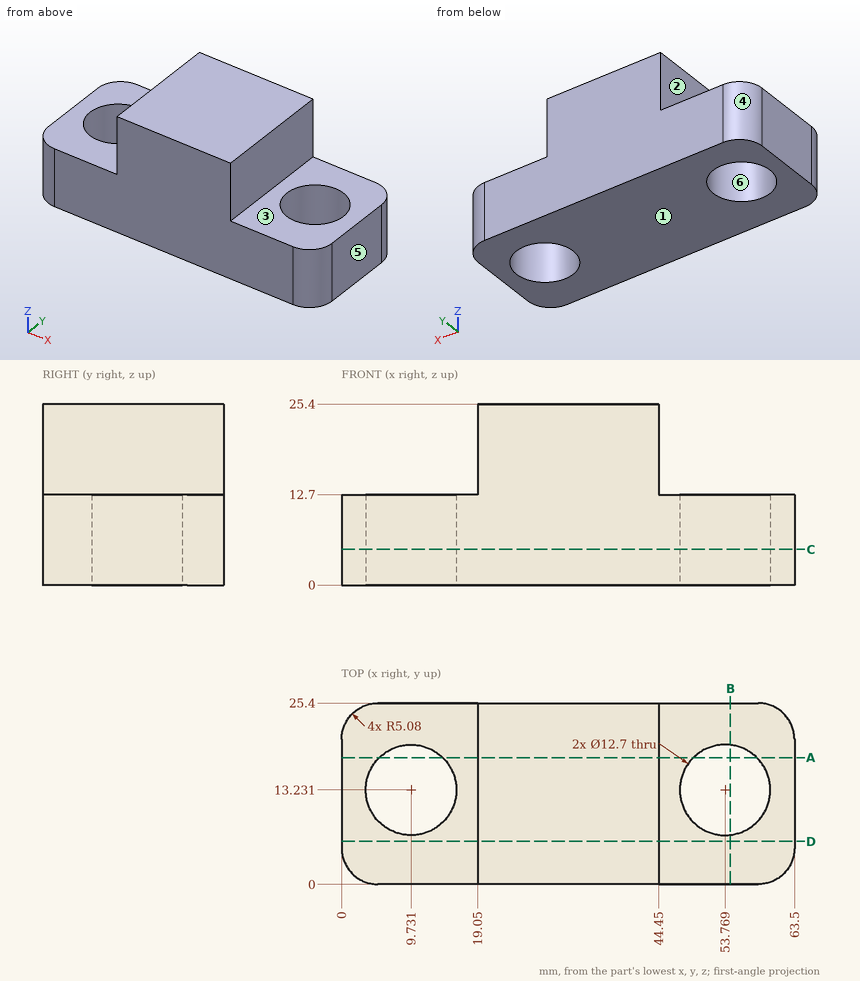
Input: dimensioned drawing with shaded views. Units: mm. Origin: part minimum x, y, z. A direction names the side the tool comes from. Coordinates: 2 decimals unless noted, no trailing zeros. Order: outer loops, then holes, each group sorted by start corner. A loop starts at its lowest first (then second) coordinate and runs counter-clockwise, first axis right, second up. Notation, with made-up numbers: (28.5, -15) - (49.5, -15) arc R20 ccw to (49.5, 13) - close; hole circle Ø6 at (30, 34). An arc over 180 degrees is marked (long way). Return JSON: item names as keys, results as strings. Group by question number.
1. Pull-direction query (Y, two-part tool) for the marked faces 4, 5 and 6; classes: pulls with the +Y half, pulls with the -Y half, needs draft (parallel to the pull), parting line crosses it, or undercut.
2. Pin query (flat end, axial travel): pin 1 (4 mm diameter, centred on y = 10.5, z = 18, fed in from +X); pin 2 (1 mm diameter, centred on x = 53, z = 13.5, fed in from -Y); pin 3 (12 mm diameter, centred on x = 47, y = 11.5, fed in from +Z); pin 4 (10 mm diameter, centred on y = 13, z = 21, fed in from -X). Return the tip coordinate at first contact, or that it passes through.
3. Cut plane B-B (x = 54.5). Output: boundary loops of the cut face in (y, z), plus the area to 3 significant figures.
4. Material intervals for line 1 along Z through (x, y) = (48, 22); line 2 along X through (y, z) = (11.5, 10.5); line 3 along X through (y, z) = (9.75, 10.75), sorted ascending. Write a range as [from, to].
5. Cut plane C-C (z = 5). Output: boundary loops of the cut face in (x, y), plus the area to 3 significant figures.
6. Set-up query: the marked faces 1, 2 and 3. Return all of +Z, -Z, +X, -X, +Y, -Y with unobstructed straight access to the full face (end or side cutting, diameter ignored); none if empty.
7. Cut plane A-A (y = 17.75). Output: boundary loops of the cut face in (x, z).
8. Cut plane D-D (y = 6). Output: boundary loops of the cut face in (x, z), plus the area to 3 significant figures.
Resolved:
{
 "1": {"face 4": "pulls with the +Y half", "face 5": "needs draft", "face 6": "undercut"},
 "2": {"pin 1": "stops at x = 44.45", "pin 2": "passes through", "pin 3": "stops at z = 25.4", "pin 4": "stops at x = 19.05"},
 "3": {"outline": "(0, 0) - (6.92, 0) - (6.92, 12.7) - (0, 12.7) - close; (19.54, 0) - (25.4, 0) - (25.4, 12.7) - (19.54, 12.7) - close", "area": "162 mm²"},
 "4": {"line 1": "z = [0, 12.7]", "line 2": "x = [0, 3.62], [15.84, 47.66], [59.88, 63.5]", "line 3": "x = [0, 4.42], [15.04, 48.46], [59.08, 63.5]"},
 "5": {"outline": "(0, 5.08) arc R5.08 ccw to (5.08, 0) - (58.42, 0) arc R5.08 ccw to (63.5, 5.08) - (63.5, 20.32) arc R5.08 ccw to (58.42, 25.4) - (5.08, 25.4) arc R5.08 ccw to (0, 20.32) - close; hole circle Ø12.7 at (9.73, 13.23); hole circle Ø12.7 at (53.77, 13.23)", "area": "1,340 mm²"},
 "6": {"face 1": "-Z, +X, -X, +Y, -Y", "face 2": "+Z, -X, +Y, -Y", "face 3": "+Z, +X, +Y, -Y"},
 "7": {"outline": "(0, 0) - (5.27, 0) - (5.27, 12.7) - (0, 12.7) - close; (14.19, 0) - (49.31, 0) - (49.31, 12.7) - (44.45, 12.7) - (44.45, 25.4) - (19.05, 25.4) - (19.05, 12.7) - (14.19, 12.7) - close; (58.23, 0) - (63.5, 0) - (63.5, 12.7) - (58.23, 12.7) - close"},
 "8": {"outline": "(0, 0) - (63.5, 0) - (63.5, 12.7) - (44.45, 12.7) - (44.45, 25.4) - (19.05, 25.4) - (19.05, 12.7) - (0, 12.7) - close", "area": "1,130 mm²"}
}
